from build123d import *

# Parameters (mm, degrees)
SKETCH2_W                      = 3
SKETCH2_H                      = 10.78
BOSS_EXTRUDE2_DEPTH            = 3
HOLE_FOR_M3_300_SC_NUTS_SP_1_D = 4.22


with BuildPart() as part:
    # Sketch2 → Boss-Extrude2 (new body)
    with BuildSketch(Plane(origin=(0, 0, 0), x_dir=(0, 0, -1), z_dir=(1, 0, 0))):
        Polygon((0, 0), (2.89, 0), (2.89, 5), (2.5, 5), (2.5, 7), (2.89, 7), (2.89, 10), (7.11, 10), (7.11, 7), (7.5, 7), (7.5, 5), (7.11, 5), (7.11, 0), (17.11, 0), (17.11, -3), (47.89, -3), (47.89, 0), (57.89, 0), (57.89, 5), (57.5, 5), (57.5, 7), (57.89, 7), (57.89, 10), (62.11, 10), (62.11, 7), (62.5, 7), (62.5, 5), (62.11, 5), (62.11, 0), (72.11, 0), (72.11, -3), (102.89, -3), (102.89, 0), (112.89, 0), (112.89, 5), (112.5, 5), (112.5, 7), (112.89, 7), (112.89, 10), (117.11, 10), (117.11, 7), (117.5, 7), (117.5, 5), (117.11, 5), (117.11, 0), (120, 0), (120, 50), (0, 50), align=None)
        with Locations((115, 30)):
            Rectangle(SKETCH2_W, SKETCH2_H, mode=Mode.SUBTRACT)
        with Locations((5, 30)):
            Rectangle(SKETCH2_W, SKETCH2_H, mode=Mode.SUBTRACT)
    extrude(amount=BOSS_EXTRUDE2_DEPTH)

    # Hole for M3 300® SC Nuts (SP)1 (through all)
    with Locations(Plane(origin=(3, 0, 0), x_dir=(0, 0, -1), z_dir=(1, 0, 0))):
        with Locations((5, 42.695), (5, 17.305), (115, 42.695), (115, 17.305)):
            Hole(HOLE_FOR_M3_300_SC_NUTS_SP_1_D / 2)


solid = part.part
Input: part model. Units: mm. Frame: model coordinates. A direction names the side the tool comes from. Give positions to 0.01 mm unless a question says otherwise; leave off trailing zeros. Order: outer loops, then holes, each group sorted by start corner. A loop starts at its lowest first (then second) coordinate and runs counter-clockwise, first axis right, second up. Notation, with made-up numbers: M 46.25,20.25 L 65.25,20.25 A28 ccw 65.25,42.25 Z; hole C 61.25,49.5 d3. An arc over 180 degrees is marked long. Answer as a JSON object with one key per item and string values.
1. First-contact query: P1, Ø0.9, axis at x = 1, z = -115.5, coming from the -Y side; P2, Ø1, axis at x = 0.5, y = 10, coming from the +Z side. Flat tips, straight axial feed; report the tip coordinate or a pass-through.
Result sheet:
{"P1": "y = 10", "P2": "z = 0"}
2. Ray query, line 1 (Z direction, x = 1.05, y = 27.5); line 2 (Y direction, x = 2.3, z = -115) (3 decimals); line 3 (Z direction, x = 2.95, y = 42.5). Return the intervals inside material, ascending. Write a range as [from, to].
Result sheet:
{"line 1": "[-120, -116.5], [-113.5, -6.5], [-3.5, 0]", "line 2": "[10, 15.195], [19.415, 24.61], [35.39, 40.585], [44.805, 50]", "line 3": "[-120, -117.1], [-112.9, -7.1], [-2.9, 0]"}
3. Pull-direction query (Z, two-part tool) for faces 1 (the flat face through (1, 50, -61)), 2 (the flat face through (1, -2, -102.89)), 3 (the flat face through (1, 2, -112.89)), 4 (the flat face through (1, 9, -7.11)); classes: +Z half, -Z half, draft (parallel to the pull), parting line (faces both ways), or undercut.
Result sheet:
{"face 1": "draft", "face 2": "-Z half", "face 3": "undercut", "face 4": "undercut"}
4. Reachability of faces 5 (the flat face through (1, 24.61, -5)), 6 (the flat face through (1, -1, -17.11)), 7 (the flat face through (1, 2, -2.89)), 8 (the flat face through (1, 25, 0)) from +Z, -Z, +X, -X, +Y, -Y: full face, straight path, thin tool, end or side. Return the list, or none.
Result sheet:
{"face 5": "+X, -X", "face 6": "+Z, +X, -X, -Y", "face 7": "+X, -X, -Y", "face 8": "+Z, +X, -X, +Y, -Y"}
5. Cut plane A-A, the plane z = -115. Output: boundary loops of the cut face in (x, y) (3 decimals).
Result sheet:
{"outline": "M 0,10 L 3,10 L 3,15.195 L 0,15.195 Z; M 0,19.415 L 3,19.415 L 3,24.61 L 0,24.61 Z; M 0,35.39 L 3,35.39 L 3,40.585 L 0,40.585 Z; M 0,44.805 L 3,44.805 L 3,50 L 0,50 Z"}
6. Cut plane C-C, the plane x = 1.25. State how many separate pieces and enclosed holes the cut face has, and give its area (3 significant figures).
Result sheet:
{"separate pieces": "1", "enclosed holes": "6", "area": "5,930 mm²"}
7. Cut plane B-B, the plane z = -49. Output: boundary loops of the cut face in (x, y).
Result sheet:
{"outline": "M 0,0 L 3,0 L 3,50 L 0,50 Z"}
